```python
from build123d import *

# Parameters (mm, degrees)
SKETCH1_W           = 42
SKETCH1_H           = 58
BOSS_EXTRUDE1_DEPTH = 3
SKETCH2_W           = 3
SKETCH2_H           = 7.199999996
SKETCH2_H_2         = 7.35
CUT_EXTRUDE1_DEPTH  = 3
SKETCH3_W           = 42
SKETCH3_H           = 1.5
CUT_EXTRUDE2_DEPTH  = 4


with BuildPart() as part:
    # Sketch1 → Boss-Extrude1 (new body)
    with BuildSketch(Plane.XY):
        with Locations((21, 29)):
            Rectangle(SKETCH1_W, SKETCH1_H)
    extrude(amount=BOSS_EXTRUDE1_DEPTH)

    # Sketch2 → Cut-Extrude1 (cut)
    with BuildSketch(Plane.XY.offset(3)):
        with Locations((40.5, 47.24818585)):
            Rectangle(SKETCH2_W, SKETCH2_H)
        with Locations((40.5, 32.848185857)):
            Rectangle(SKETCH2_W, SKETCH2_H)
        with Locations((1.5, 47.24818585)):
            Rectangle(SKETCH2_W, SKETCH2_H)
        with Locations((1.5, 32.848185857)):
            Rectangle(SKETCH2_W, SKETCH2_H)
        with Locations((1.5, 11.023185866)):
            Rectangle(SKETCH2_W, SKETCH2_H_2)
        with Locations((40.5, 11.023185866)):
            Rectangle(SKETCH2_W, SKETCH2_H_2)
    extrude(amount=-CUT_EXTRUDE1_DEPTH, mode=Mode.SUBTRACT)

    # Sketch3 → Cut-Extrude2 (cut, through all)
    with BuildSketch(Plane.XY.offset(3)):
        with Locations((21, 0.75)):
            Rectangle(SKETCH3_W, SKETCH3_H)
    extrude(amount=-CUT_EXTRUDE2_DEPTH, mode=Mode.SUBTRACT)


solid = part.part
```
Read the model definition and answer for the solid it produces. Units are mm, in the model's axes. A direction names the side the tool comes from. Coordinates: 2 decimals unless noted, no trailing zeros. Loops run counter-clockwise (first coordinate to the right, second up) from the corner with the lowest first, then second, coordinate; pieces in that order, holes last.
(1) A tool of negligible diameter and unlimited length cuts with its end or side. For faces 5 (the face through (0, 22, 1)), 6 (the face through (1, 36.448, 2)), 7 (the face through (39, 33, 2)), from which of +Z, -Z, +X, -X, +Y, -Y can it reach the whole face along a straight path? Write none if from no direction.
Solution:
face 5: +Z, -Z, -X, +Y, -Y
face 6: +Z, -Z, -X
face 7: +Z, -Z, +X
(2) The mould has two halves that part along Y. Classify faces 1 (the face through (40, 29.248, 2)), 2 (the face through (21, 30, 3)), 3 (the face through (21, 58, 1)), 4 (the face through (21, 1.5, 2)): released by +Y, released by -Y, zero draft, split by the parting line, or undercut.
Solution:
face 1: undercut
face 2: zero draft
face 3: released by +Y
face 4: released by -Y
(3) Flat-ended cylindrical pins translate along their axes: pin 1 Ø0.9 at (y, z) = (9.5, 1) entering from +X; pin 2 Ø1 at (y, z) = (44.5, 2) entering from -X. Find the tip coordinate at first contact, or state that the pin passes through.
Solution:
pin 1: stops at x = 39
pin 2: stops at x = 3
(4) The part is cut by section A-A (z = 1.1). Determine the outline of the cut face in (x, y).
Solution:
outline: (0, 1.5) - (42, 1.5) - (42, 7.35) - (39, 7.35) - (39, 14.7) - (42, 14.7) - (42, 29.25) - (39, 29.25) - (39, 36.45) - (42, 36.45) - (42, 43.65) - (39, 43.65) - (39, 50.85) - (42, 50.85) - (42, 58) - (0, 58) - (0, 50.85) - (3, 50.85) - (3, 43.65) - (0, 43.65) - (0, 36.45) - (3, 36.45) - (3, 29.25) - (0, 29.25) - (0, 14.7) - (3, 14.7) - (3, 7.35) - (0, 7.35) - close
(5) Consider line 1 along X through (y, z) = (31.5, 0.75). Determine where the line is inside the solid, lowest interval first.
Solution:
line 1: x = 3 to 39
